Read the model definition and answer for the solid it produces. Units are mm, in the model's axes. A direction names the side the tool comes from. Give positions to 0.01 mm unless a question says otherwise; leave off trailing zeros. Order: outer loops, then holes, each group sorted by start corner. A loop starts at its lowest first (then second) coordinate and runs counter-clockwise, first axis right, second up. Notation, with made-up numbers: (67, -25) - (101, -25) arc R22 ccw to (101, 2) - close; hole circle Ø9 at (77, -38.5). An arc over 180 degrees is marked (long way). Write each question's results on one line, items separated by ' | '.
Autodesk Inventor part; units mm, degrees
ref_plane "YZ Plane" through (0, 0, 0) normal (1, 0, 0) x (0, 1, 0)
ref_plane "XZ Plane" through (0, 0, 0) normal (0, 1, 0) x (-1, 0, 0)
ref_plane "XY Plane" through (0, 0, 0) normal (0, 0, 1) x (1, 0, 0)
sketch "Sketch4" plane through (0, 0, 0) normal (0, 0, 1) x (1, 0, 0)
  line L0 (10.9923, 14.2423) -> (-9.6452, 14.2423)
  line L1 (11.786, 15.036) -> (11.786, 25.9263)
  line L2 (13.3735, 26.9423) -> (11.786, 26.9423)
  line L3 (-10.439, 15.036) -> (-10.439, 25.9263)
  line L4 (-10.439, 26.9423) -> (-12.0265, 26.9423)
  arc A0 (-10.439, 15.036) -> (-9.6452, 14.2423) centre (-9.6452, 15.036) ccw
  arc A1 (10.9923, 14.2423) -> (11.786, 15.036) centre (10.9923, 15.036) ccw
  arc A2 (11.786, -24.6515) -> (10.9923, -23.8577) centre (10.9923, -24.6515) ccw
  line L5 (-9.6452, -23.8577) -> (10.9923, -23.8577)
  arc A3 (-9.6452, -23.8577) -> (-10.439, -24.6515) centre (-9.6452, -24.6515) ccw
  line L6 (-10.439, -24.6515) -> (-10.439, -36.5577)
  line L7 (11.786, -24.6515) -> (11.786, -36.5577)
  line L8 (11.786, 26.9423) -> (11.786, 25.9263)
  line L9 (-10.439, 26.9423) -> (-10.439, 25.9263)
  line L10 (11.786, -24.6515) -> (-10.439, -24.6515)
  line L11 (11.786, 15.036) -> (-10.439, 15.036)
  line L12 (11.786, 26.9423) -> (11.532, 26.9423)
  line L13 (11.532, 26.9423) -> (11.532, 15.036)
  line L14 (-10.439, 26.9423) -> (-10.185, 26.9423)
  line L15 (-10.185, 26.9423) -> (-10.185, 15.036)
  line L16 (11.532, 26.9423) -> (-10.185, 26.9423)
  line L17 (11.786, -24.6515) -> (11.532, -24.6515)
  line L18 (11.532, -24.6515) -> (11.532, -36.5577)
  line L19 (11.532, -36.5577) -> (11.786, -36.5577)
  line L20 (11.786, -36.5577) -> (11.786, -24.6515)
  line L21 (-10.439, -24.6515) -> (-10.185, -24.6515)
  line L22 (-10.185, -24.6515) -> (-10.185, -36.5577)
  line L23 (-10.185, -36.5577) -> (-10.439, -36.5577)
  line L24 (-10.439, -36.5577) -> (-10.439, -24.6515)
  line L25 (11.532, -36.5577) -> (-10.439, -36.5577)
  line L26 (0, 14.2423) -> (0, -23.8577)
  point P0 (0, 0)
  dimension "d5" = 22.225
  dimension "d6" = 0.254
  dimension "d7" = 0.254
  dimension "d14" = 38.1
extrude "Extrusion2" add sketch "Sketch4" against normal blind 25.4 contours L11 L15 L16 L13 | L18 L25 L22 L10
sketch "Sketch5" plane through (11.532, -36.5577, 0) normal (1, 0, 0) x (0, 0, -1)
  point P0 (0, 36.5577)
sketch "Sketch6" plane through (11.532, -36.5577, 0) normal (1, 0, 0) x (0, 0, -1)
  line L0 (0, 51.5938) -> (0, 63.5)
  line L1 (0, 51.5938) -> (25.4, 51.5938)
  line L2 (25.4, 63.5) -> (25.4, 51.5938)
  line L3 (0, 63.5) -> (25.4, 63.5)
  line L4 (0, 0) -> (0, 11.9062)
  line L5 (0, 0) -> (25.4, 0)
  line L6 (25.4, 11.9062) -> (25.4, 0)
  line L7 (0, 11.9062) -> (25.4, 11.9062)
  line L8 (25.4, 63.5) -> (25.4, 57.15)
  line L9 (25.4, 57.15) -> (19.05, 57.15)
  line L10 (25.4, 0) -> (25.4, 6.35)
  line L11 (25.4, 6.35) -> (19.05, 6.35)
  line L12 (25.4, 62.484) -> (25.4, 51.5938)
  line L13 (37.3758, 42.3425) -> (37.3758, 45.2438)
  line L14 (37.3758, 63.5) -> (25.4, 63.5)
  line L15 (37.3758, 0) -> (25.4, 0)
  line L16 (25.4, 63.5) -> (37.3758, 63.5)
  line L17 (46.355, 51.9072) -> (46.355, 11.5928)
  line L18 (37.3758, 0) -> (25.4, 0)
  line L19 (25.4, 51.5938) -> (31.0258, 51.5938)
  line L20 (25.4, 11.9062) -> (31.0258, 11.9062)
  arc A0 (37.3758, 45.2438) -> (31.0258, 51.5938) centre (31.0258, 45.2438) ccw
  line L21 (46.355, 51.9072) -> (46.355, 50.8)
  arc A1 (46.355, 50.8) -> (37.3758, 63.5) centre (33.6671, 51.3536) ccw
  arc A2 (31.0258, 11.9062) -> (37.3758, 18.2562) centre (31.0258, 18.2562) ccw
  line L22 (46.355, 11.5928) -> (46.355, 12.7)
  arc A3 (37.3758, 0) -> (46.355, 12.7) centre (33.6671, 12.1464) ccw
  line L23 (37.3758, 42.3425) -> (37.3758, 18.2562)
  line L24 (25.4, 6.35) -> (19.05, 6.35)
  circle A4 centre (19.05, 57.15) radius 2.3241
  circle A5 centre (6.35, 57.15) radius 2.3241
  line L25 (25.4, 6.35) -> (19.05, 6.35)
  circle A6 centre (19.05, 6.35) radius 2.3241
  line L26 (19.05, 6.35) -> (6.35, 6.35)
  circle A7 centre (6.35, 6.35) radius 2.3241
  point P0 (0, 36.5577)
  dimension "d15" = 6.35
  dimension "d16" = 6.35
  dimension "d17" = 6.35
  dimension "d35" = 4.6482
  dimension "d36" = 4.6482
  dimension "d37" = 12.7
  dimension "d38" = 4.6482
extrude "Extrusion3" add sketch "Sketch6" against normal up to surface (21.717 mm away) contours L2 L14 A1 L17 A3 L15 L6 L20 A2 L23 L13 A0 L19
extrude "Extrusion4" cut sketch "Sketch6" along normal through all both and the other way through all contours A6 L26 L11 | L11 L26 A6 | A4 | A5 | A7
fillet "Fillet1" radius 13.97 2 edges at (0.6735, 26.9423, -37.3758) (0.6735, -36.5577, -37.3758)
fillet_without_effect "Fillet2"
sketch "Sketch7" plane through (11.532, 15.036, 0) normal (1, 0, 0) x (0, 0, -1)
  arc A0 (37.3758, -6.35) -> (31.0258, 0) centre (31.0258, -6.35) ccw
  line L0 (0, 0) -> (31.0258, 0)
  line L1 (0, 11.9063) -> (32.385, 11.9063)
  arc A1 (46.355, -2.0638) -> (32.385, 11.9063) centre (32.385, -2.0637) ccw
  line L2 (46.355, -37.6238) -> (46.355, -2.0638)
  arc A2 (31.0258, -39.6875) -> (37.3758, -33.3375) centre (31.0258, -33.3375) ccw
  line L3 (37.3758, -6.35) -> (37.3758, -33.3375)
  arc A3 (32.385, -51.5938) -> (46.355, -37.6238) centre (32.385, -37.6238) ccw
  line L4 (0, -39.6875) -> (31.0258, -39.6875)
  line L5 (0, -51.5938) -> (32.385, -51.5938)
  line L6 (37.3758, -6.35) -> (37.3758, -11.43)
  line L7 (37.3758, -11.43) -> (24.169, -11.43)
  line L8 (25.4, 10.8903) -> (25.4, 0)
  line L9 (37.3758, -11.43) -> (33.5658, -11.43)
  line L10 (25.4, 0) -> (33.5658, -11.43)
  line L11 (33.5658, -11.43) -> (37.3758, -16.763)
  line L12 (37.3758, -16.763) -> (46.355, -16.763)
  line L13 (25.4, 0) -> (25.4, 11.9063)
  line L14 (25.4, 11.9063) -> (46.355, -16.763)
  arc A4 (32.385, -51.5938) -> (46.355, -37.6238) centre (32.385, -37.6238) ccw
  line L15 (46.355, -37.6238) -> (46.355, -2.0638)
  arc A5 (46.355, -2.0638) -> (32.385, 11.9063) centre (32.385, -2.0637) ccw
  line L16 (0, 11.9063) -> (32.385, 11.9063)
  line L17 (0, 0) -> (0, 11.9063)
  line L18 (0, 0) -> (31.0258, 0)
  arc A6 (37.3758, -6.35) -> (31.0258, 0) centre (31.0258, -6.35) ccw
  line L19 (37.3758, -6.35) -> (37.3758, -33.3375)
  arc A7 (31.0258, -39.6875) -> (37.3758, -33.3375) centre (31.0258, -33.3375) ccw
  line L20 (0, -39.6875) -> (31.0258, -39.6875)
  line L21 (0, -51.5938) -> (0, -39.6875)
  line L22 (0, -51.5938) -> (32.385, -51.5938)
  circle A8 centre (19.05, -45.2438) radius 2.3241
  circle A9 centre (6.35, 5.5563) radius 2.3241
  circle A10 centre (6.35, -45.2438) radius 2.3241
  circle A11 centre (19.05, 5.5563) radius 2.3241
  line L23 (46.355, -37.6238) -> (43.4517, -37.6238)
  point P0 (0, -15.036)
  point P1 (36.7783, -3.6607)
  point P2 (35.3345, -1.6854)
  dimension "d43" = 5.08
  dimension "d44" = 3.81
extrude "Extrusion5" add sketch "Sketch7" against normal up to surface (21.717 mm away) contours L3 L7 L10 L0 A0 L14 | L3 L11 L7
extrude "Extrusion6" cut sketch "Sketch7" along normal through all both and the other way through all contours A0 L14 L1 A1 L2
fillet "Fillet3" radius 6.35 2 edges at (0.6735, 26.9423, -25.4) (0.6735, -1.727, -46.355)
fillet "Fillet4" radius 6.35 1 edges at (0.6735, -1.727, -37.3758)
properties part number "Front_support_Intake"
(1) Consider probe 1 along Y at (x, z) = (1, -19.05); probe 2 along Y at (x, z) = (2.75, -16); probe 3 along Y at (x, z) = (9.5, -4.5). Determine where each line is inside the solid, lowest interval first. Write a range as [from, to].
Conclusion:
probe 1: [-36.56, -32.53], [-27.88, -24.65], [15.04, 18.27], [22.92, 26.94] | probe 2: [-36.56, -24.65], [15.04, 26.94] | probe 3: [-36.56, -31.61], [-28.8, -24.65], [15.04, 19.19], [22, 26.94]
(2) Section A-A (z = -6.35) is taken. Give the vertices of the cut face in (x, y) (1 decimal), plus the area to 3 significant figures.
Conclusion:
outline: (-10.2, -36.6) - (11.5, -36.6) - (11.5, -32.5) - (-10.2, -32.5) - close; (-10.2, -27.9) - (11.5, -27.9) - (11.5, -24.7) - (-10.2, -24.7) - close; (-10.2, 15) - (11.5, 15) - (11.5, 18.3) - (-10.2, 18.3) - close; (-10.2, 22.9) - (11.5, 22.9) - (11.5, 26.9) - (-10.2, 26.9) - close | area: 315 mm^2
(3) Section B-B (z = -28.5) is taken. Give the vertices of the cut face in (x, y) (1 decimal).
Conclusion:
outline: (-10.2, -36.6) - (11.5, -36.6) - (11.5, -24.7) - (-10.2, -24.7) - close; (-10.2, 10.7) - (11.5, 10.7) - (11.5, 22.7) - (-10.2, 22.7) - close
(4) The mould has two halves that part along Z. Classify faces 1 (the face through (0.826, -32.477, -18.546)), 2 (the face through (1, -13, -46.355)), 3 (the face through (-10.185, -11, -38)): pulls with the +Z half, pulls with the -Z half, needs draft (parallel to the pull), parting line crosses it, or undercut.
Conclusion:
face 1: undercut | face 2: pulls with the -Z half | face 3: needs draft
(5) Each of these flat-tipped pins is pushed along its axis until it touches: pin 1 (1 mm diameter, centred on x = 0.5, y = -3.5, fed in from +Z); pin 2 (3 mm diameter, centred on x = -1.5, y = 18, fed in from -Z); pin 3 (1 mm diameter, centred on x = -4.5, z = -37.5, fed in from +Y). Where does it stop, or does it pass through?
Conclusion:
pin 1: z = -37.33 | pin 2: z = -33.03 | pin 3: y = 11.07
(6) For faces 4 (the face through (0.5, 12.3, -36.1)), 5 (the face through (0.826, -22.841, -35.466)), determine the directions among +Z, -Z, +X, -X, +Y, -Y from which every point of the face is accessible in a straight line to the end or side of a thin tool.
Conclusion:
face 4: -Z, +X, -X, +Y | face 5: +Z, +X, -X
(7) Section D-D (x = 7.75) is taken. State how many separate pieces and enclosed holes the cut face has, plus the area to 3 significant figures.
Conclusion:
separate pieces: 1 | enclosed holes: 4 | area: 1,160 mm^2
